Autodesk Inventor part; units mm, degrees
ref_plane "Work Plane1" through (32.5, 0, 0) normal (-1, 0, 0) x (0, 0, 1)
ref_plane "YZ Plane" through (0, 0, 0) normal (1, 0, 0) x (0, 1, 0)
ref_plane "XZ Plane" through (0, 0, 0) normal (0, 1, 0) x (-1, 0, 0)
sketch "Sketch1" plane through (0, 0, 0) normal (1, 0, 0) x (0, 1, 0)
  circle A0 centre (0, 0) radius 1.75
  circle A1 centre (15, 0) radius 1.75
  line L0 (15, 0) -> (0, 0) construction
  line L1 (15, 0) -> (15, 51.4) construction
  line L2 (0, 0) -> (0, 51.4) construction
  circle A2 centre (0, 51.4) radius 1.75
  circle A3 centre (15, 51.4) radius 1.75
  line L3 (15, 25.7) -> (15.4, 25.7) construction
  line L4 (20, 57.4) -> (-5, 57.4)
  line L5 (-5, 57.4) -> (-5, 45.4)
  line L6 (-5, 45.4) -> (20, 45.4)
  line L7 (20, 45.4) -> (20, 57.4)
  line L8 (20, 6) -> (-5, 6)
  line L9 (-5, 6) -> (-5, -6)
  line L10 (-5, -6) -> (20, -6)
  line L11 (20, -6) -> (20, 6)
  line L12 (7.5, 45.4) -> (7.5, 0) construction
  line L13 (15, 51.4) -> (20, 51.4) construction
  line L14 (15, 0) -> (20, 0)
  circle A4 centre (15.4, 25.7) radius 2.6
  line L15 (55.1, 45.7) -> (55.1, 5.7) construction
  circle A5 centre (55.1, 45.7) radius 2.6
  circle A6 centre (55.1, 5.7) radius 2.6
  line L16 (55.1, 25.7) -> (15.4, 25.7) construction
  dimension "d0" = 3.5
  dimension "d1" = 15
  dimension "d2" = 51.4
  dimension "d3" = 51.4
  dimension "d15" = 0.4
  dimension "d20" = 12
  dimension "d21" = 25
  dimension "d60" = 5.2
  dimension "d61" = 40
  dimension "d62" = 39.7
extrude "Extrusion3" add sketch "Sketch1" along normal blind 8 contours L11 L10 L9 L8 | L7 L6 L5 L4
sketch "Sketch3" plane through (0, -5, -6) normal (0, -1, 0) x (1, 0, 0)
  arc A0 (0, 51.4) -> (0, 12) centre (-22.6254, 31.7) ccw construction
  arc A1 (8, 51.4) -> (8, 12) centre (-14.6254, 31.7) ccw construction
  line L0 (0, 51.4) -> (0, 63.4)
  line L1 (0, 63.4) -> (8, 63.4)
  line L2 (8, 51.4) -> (8, 63.4)
  line L3 (0, 51.4) -> (8, 51.4)
  line L4 (0, 0) -> (0, 12)
  line L5 (0, 12) -> (8, 12)
  line L6 (8, 0) -> (8, 12)
  line L7 (0, 0) -> (8, 0)
  arc A2 (8, 12) -> (8, 51.4) centre (-14.6254, 31.7) ccw
  arc A3 (0, 12) -> (0, 51.4) centre (-22.6254, 31.7) ccw
  point P0 (0, 6)
  dimension "d24" = 60
extrude "Extrusion4" add sketch "Sketch3" against normal up to surface (25 mm away) contours L3 A2 L5 A3
ref_plane "Work Plane1" through (32.5, 0, 0) normal (-1, 0, 0) x (0, 0, 1)
sketch "Sketch4" plane through (32.5, 0, 0) normal (-1, 0, 0) x (0, 0, 1)
  circle A0 centre (25.7, 15.4) radius 2.6
  circle A1 centre (45.7, 55.1) radius 2.6
  circle A2 centre (5.7, 55.1) radius 2.6
  line L0 (25.7, 15) -> (25.7, 15.4) construction
  line L1 (50.7, 10.4) -> (0.7, 10.4)
  line L2 (0.7, 10.4) -> (0.7, 60.1)
  line L3 (0.7, 60.1) -> (50.7, 60.1)
  line L4 (50.7, 60.1) -> (50.7, 10.4)
  line L5 (28.3, 10.4) -> (28.3, 15.4)
  line L6 (23.1, 10.4) -> (23.1, 15.4)
  point P0 (25.7, 55.1)
  dimension "d67" = 5
  dimension "d68" = 5
  dimension "d69" = 5
  dimension "d70" = 5
extrude "Extrusion5" add sketch "Sketch4" along normal blind 10 contours A0 L6 L1 L2 L3 L4 L5
sketch "Sketch8" plane through (8, 0, 0) normal (1, 0, 0) x (0, 0, -1)
  circle A0 centre (-51.4, 0) radius 1.75
  line L0 (-54.6909, 0) -> (-53.0454, 2.85)
  line L1 (-53.0454, 2.85) -> (-49.7546, 2.85)
  line L2 (-49.7546, 2.85) -> (-48.1091, 0)
  line L3 (-48.1091, 0) -> (-49.7546, -2.85)
  line L4 (-49.7546, -2.85) -> (-53.0454, -2.85)
  line L5 (-53.0454, -2.85) -> (-54.6909, 0)
  circle A1 centre (-51.4, 15) radius 1.75
  line L6 (-54.6909, 15) -> (-53.0454, 17.85)
  line L7 (-53.0454, 17.85) -> (-49.7546, 17.85)
  line L8 (-49.7546, 17.85) -> (-48.1091, 15)
  line L9 (-48.1091, 15) -> (-49.7546, 12.15)
  line L10 (-49.7546, 12.15) -> (-53.0454, 12.15)
  line L11 (-53.0454, 12.15) -> (-54.6909, 15)
  line L12 (-3.2909, 0) -> (-1.6454, 2.85)
  line L13 (-1.6454, 2.85) -> (1.6454, 2.85)
  line L14 (1.6454, 2.85) -> (3.2909, 0)
  line L15 (3.2909, 0) -> (1.6454, -2.85)
  line L16 (1.6454, -2.85) -> (-1.6454, -2.85)
  line L17 (-1.6454, -2.85) -> (-3.2909, 0)
  circle A2 centre (0, 15) radius 1.75
  line L18 (-3.2909, 15) -> (-1.6454, 17.85)
  line L19 (-1.6454, 17.85) -> (1.6454, 17.85)
  line L20 (1.6454, 17.85) -> (3.2909, 15)
  line L21 (3.2909, 15) -> (1.6454, 12.15)
  line L22 (1.6454, 12.15) -> (-1.6454, 12.15)
  line L23 (-1.6454, 12.15) -> (-3.2909, 15)
  circle A3 centre (0, 0) radius 1.75
  dimension "d54" = 5.7
extrude "Extrusion7" cut sketch "Sketch8" against normal blind 3.5 contours A0 | L0 L1 L2 L3 L4 L5 | A1 | L6 L7 L8 L9 L10 L11 | L12 L13 L14 L15 L16 L17 | A2 | L18 L19 L20 L21 L22 L23 | A3
sketch "Sketch10" plane through (22.5, 0, 0) normal (-1, 0, 0) x (0, 0, 1)
  line L0 (50.7, 10.4) -> (50.7, 60.1)
  line L1 (50.7, 50.1) -> (40.7, 50.1)
  line L2 (40.7, 50.1) -> (40.7, 35.25)
  line L3 (40.7, 10.4) -> (50.7, 10.4)
  line L4 (50.7, 10.4) -> (50.7, 50.1)
  line L5 (0.7, 10.4) -> (50.7, 10.4)
  line L6 (0.7, 60.1) -> (0.7, 10.4)
  line L7 (10.7, 10.4) -> (0.7, 10.4)
  line L8 (0.7, 10.4) -> (0.7, 50.1)
  line L9 (0.7, 50.1) -> (10.7, 50.1)
  line L10 (10.7, 50.1) -> (10.7, 35.25)
  line L11 (40.7, 30.25) -> (10.7, 30.25) construction
  line L12 (25.7, 35.25) -> (25.7, 25.25) construction
  line L13 (40.7, 35.25) -> (10.7, 35.25)
  line L14 (40.7, 25.25) -> (10.7, 25.25)
  line L15 (10.7, 30.25) -> (0.7, 30.25) construction
  circle A0 centre (5.7, 55.1) radius 2.6
  line L16 (10.7, 25.25) -> (10.7, 10.4)
  line L17 (10.7, 35.25) -> (10.7, 25.25) construction
  line L18 (40.7, 35.25) -> (40.7, 25.25) construction
  line L19 (40.7, 25.25) -> (40.7, 10.4)
  point P0 (0, 0)
  point P1 (25.7, 30.25)
  dimension "d71" = 10
  dimension "d72" = 5
sketch "Sketch13" plane through (0, 0, 0) normal (-1, 0, 0) x (0, 0, 1)
  line L0 (45.4, 20) -> (57.4, 20)
  line L1 (57.4, -5) -> (45.4, -5)
  line L2 (6, -5) -> (45.4, -5)
  line L3 (35.4, 5) -> (16, 5)
  line L4 (-6, 20) -> (6, 20)
  line L5 (6, 20) -> (16, 20)
  line L6 (6, 20) -> (45.4, 20)
  line L7 (16, 20) -> (16, 15)
  line L8 (16, 15) -> (35.4, 15)
  line L9 (35.4, 15) -> (35.4, 20)
  line L10 (35.4, 20) -> (45.4, 20)
  line L11 (45.4, -5) -> (45.4, 20)
  line L12 (45.4, 20) -> (45.4, 0)
  line L13 (35.4, 5) -> (35.4, 0)
  line L14 (35.4, 0) -> (45.4, 0)
  line L15 (6, 20) -> (6, 0)
  line L16 (6, 20) -> (6, -5)
  line L17 (6, 0) -> (16, 0)
  line L18 (16, 0) -> (16, 5)
  point P0 (0, 0)
  dimension "d83" = 10
  dimension "d84" = 5
  dimension "d85" = 10
loft "Loft3" add profiles "Sketch10", "Sketch13" contours L3 L19 L14 L16 L5 L6 L9 L10 L13 L2 L1 L0 / L15 L5 L7 L8 L9 L6 L11 L14 L13 L3 L18 L17
sketch "Sketch14" plane through (0, -5, -6) normal (0, -1, 0) x (1, 0, 0)
  arc A0 (0, 12) -> (0, 51.4) centre (-22.6254, 31.7) ccw
  circle A1 centre (-22.6254, 31.7) radius 30
  point P0 (0, 6)
  point P1 (0, 51.4)
  point P2 (0, 12)
extrude "Extrusion10" cut sketch "Sketch14" against normal through all
sketch "Sketch15" plane through (32.5, 10.4, 0.7) normal (0, 0, -1) x (-1, 0, 0)
  line L0 (10, 0) -> (24.5, -6.7022)
  line L1 (24.5, -15.4) -> (24.5, -6.7022)
  line L2 (24.5, -6.7022) -> (24.5, -15.4)
  line L3 (24.5, -15.4) -> (10, -15.4)
  line L4 (10, 0) -> (10, 39.7)
  line L5 (10, -15.4) -> (10, 0)
  point P0 (32.5, -10.4)
extrude "Extrusion11" cut sketch "Sketch15" against normal through all
properties part number "Soporte" material "ABS Plastic"
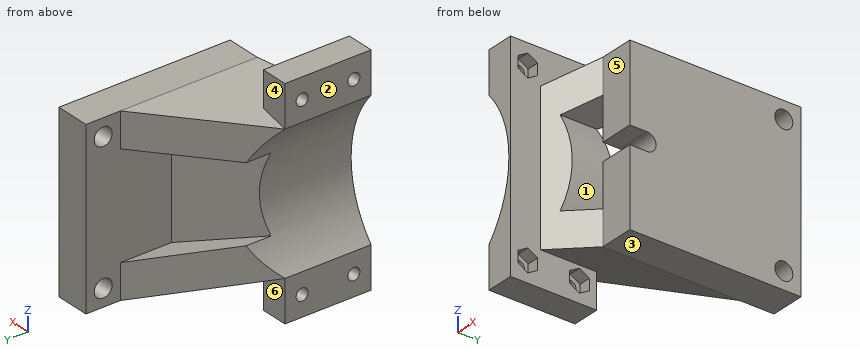
Work out the finished part from the listing and answer in its coordinate system (mm). Face numbers are marked on the shaded views. A direction names the side the tool comes from. Coordinates: 2 decimals unless noted, no trailing zeros. Loops run counter-clockwise (first coordinate to the right, second up) from the corner with the lowest first, then second, coordinate; pieces in that order, holes last. Notation, with made-up numbers: (58.25, 55.5) - (110.25, 55.5) arc R12 ccw to (110.25, 59.5) - close; hole circle Ø6 at (17.5, 12.5). An arc over 180 degrees is marked (long way). Use a Markdown table: item, result.
Item 1: The mould has two halves that part along Z. Classify the marked faces 1, 2 and 3: +Z half, -Z half, draft (parallel to the pull), parting line (faces both ways), or undercut.
Evaluation:
| item | result |
|---|---|
| face 1 | undercut |
| face 2 | draft |
| face 3 | -Z half |
Item 2: Find section B-B, the plane x = 25.5. Determine the outline of the cut face in (y, z), and give its area (3 significant figures).
Evaluation:
| item | result |
|---|---|
| outline | (10.4, 0.7) - (60.1, 0.7) - (60.1, 50.7) - (10.4, 50.7) - (10.4, 28.3) - (15.4, 28.3) arc R2.6 cw to (15.4, 23.1) - (10.4, 23.1) - close; hole circle Ø5.2 at (55.1, 5.7); hole circle Ø5.2 at (55.1, 45.7) |
| area | 2,410 mm2 |
Item 3: For the marked faces 4, 5 and 6, determine the directions among +Z, -Z, +X, -X, +Y, -Y from which every point of the face is accessible in a straight line to the end or side of a thin tool.
Evaluation:
| item | result |
|---|---|
| face 4 | +Z, -X, +Y |
| face 5 | +Z, -Z, +X, -Y |
| face 6 | -Z, -X, +Y |
Item 4: Given pin 1 Ø16.5 at (y, z) = (20.5, 21.5) entering from -X; pin 2 Ø10 at (x, y) = (25.5, 33) entering from -Z; pin 3 Ø4 at (y, z) = (16.5, 42) entering from -X, each flat-ended and moving along its own axis, determine where each tip first touches the part or whether it passes through.
Evaluation:
| item | result |
|---|---|
| pin 1 | stops at x = 4.67 |
| pin 2 | stops at z = 0.7 |
| pin 3 | stops at x = 1.15 |
Item 5: Find section A-A, the plane y = 55.1. Determine the outline of the cut face in (x, z), and give its area (3 significant figures).
Evaluation:
| item | result |
|---|---|
| outline | (22.5, 0.7) - (32.5, 0.7) - (32.5, 3.1) - (22.5, 3.1) - close; (22.5, 8.3) - (32.5, 8.3) - (32.5, 43.1) - (22.5, 43.1) - close; (22.5, 48.3) - (32.5, 48.3) - (32.5, 50.7) - (22.5, 50.7) - close |
| area | 396 mm2 |
Item 6: Find section C-C, the plane x = 3.5. State how many separate pieces and enclosed holes the cut face has, and give its area (3 significant figures).
Evaluation:
| item | result |
|---|---|
| separate pieces | 2 |
| enclosed holes | 4 |
| area | 863 mm2 |
Item 7: Consider probe 1 along Y at (x, z) = (5, -1); probe 2 along Z at (x, y) = (27, 55); probe 3 along Z at (x, y) = (2.7, 15). Determine where each line is inside the solid, lowest interval first. Write a range as from..to.
Evaluation:
| item | result |
|---|---|
| probe 1 | y = -5..-2.85, 2.85..12.15, 17.85..20 |
| probe 2 | z = 0.7..3.1, 8.3..43.1, 48.3..50.7 |
| probe 3 | z = -6..-1.75, 1.75..9.62, 41.78..49.65, 53.15..57.4 |
